Model file for the job. Use its own axes, mm. A direction names the side the tool comes from. Give positions to 0.01 mm unless a question says otherwise; leave off trailing zeros. Write each loop counter-clockwise with the first axis right and the second up, starting at its lowest first coordinate (ties: lowest second). Pieces come first, ordered by that corner, then holes. Notation, with made-up numbers: (23, -1.5) - (41, -1.5) arc R27 cw to (41, 31.5) - close; hole circle Ø10 at (-38.75, 34). An arc over 180 degrees is marked (long way). One line per item, written item: value. Start each with the question number.
(1) Cut at A-A, the plane y = -46. List the corners of the cut face in (x, z).
(2) Probe L1, parallel to Z at x = 153, y = 62.5. List the from-to ranges inside material, lowest first.
(3) Drop a flat-ended pin along its axis: P1, Ø12, axis at x = 81, y = -44.5, coming from the +Z side. Give the stop position or say it passes through.
(4) 3-axis set-ups, long thin cutter, end or side, ignore diameter. For faces 1 (the face through (12.465, -56.133, -154.93)), 2 (the face through (12.465, -56.133, 155.07)), 3 (the face through (1, 1, 160)): which of +Z, -Z, +X, -X, +Y, -Y reach the whole face in a straight line?
(5) Cut at B-B, the plane x = 0. List the corners of the cut face in (y, z).
(6) Cut at C-C, the plane x = -115. List the corners of the cut face in (y, z).
from build123d import *

# Parameters (mm, degrees)
BOSS_EXTRUDE1_DEPTH      = 150
BOSS_EXTRUDE1_DEPTH_BACK = 150
SKETCH1_W                = 400
SKETCH1_H                = 200
BOSS_EXTRUDE2_DEPTH      = 160
BOSS_EXTRUDE2_DEPTH_BACK = 160
SKETCH2_R                = 57.5


with BuildPart() as part:
    # Sketch1 → Boss-Extrude1 (new, two sides: drawn at the far end of the back side and taken through both)
    with BuildSketch(Plane.XY.offset(-BOSS_EXTRUDE1_DEPTH_BACK)):
        Rectangle(SKETCH1_W, SKETCH1_H)
    extrude(amount=BOSS_EXTRUDE1_DEPTH + BOSS_EXTRUDE1_DEPTH_BACK)

    # Sketch2 → Boss-Extrude2 (add, two sides: drawn at the far end of the back side and taken through both)
    with BuildSketch(Plane(origin=(0, 0, 0), x_dir=(-1, 0, 0), z_dir=(0, 0, -1)).offset(-BOSS_EXTRUDE2_DEPTH_BACK)):
        Circle(SKETCH2_R)
    extrude(amount=BOSS_EXTRUDE2_DEPTH + BOSS_EXTRUDE2_DEPTH_BACK)


solid = part.part
Answers follow:
1. outline: (-200, -150) - (-34.5, -150) - (-34.5, -160) - (34.5, -160) - (34.5, -150) - (200, -150) - (200, 150) - (34.5, 150) - (34.5, 160) - (-34.5, 160) - (-34.5, 150) - (-200, 150) - close
2. L1: z = -150 to 150
3. P1: stops at z = 150
4. face 1: -Z
4. face 2: +Z
4. face 3: +Z, +X, -X, +Y, -Y
5. outline: (-100, -150) - (-57.5, -150) - (-57.5, -160) - (57.5, -160) - (57.5, -150) - (100, -150) - (100, 150) - (57.5, 150) - (57.5, 160) - (-57.5, 160) - (-57.5, 150) - (-100, 150) - close
6. outline: (-100, -150) - (100, -150) - (100, 150) - (-100, 150) - close
